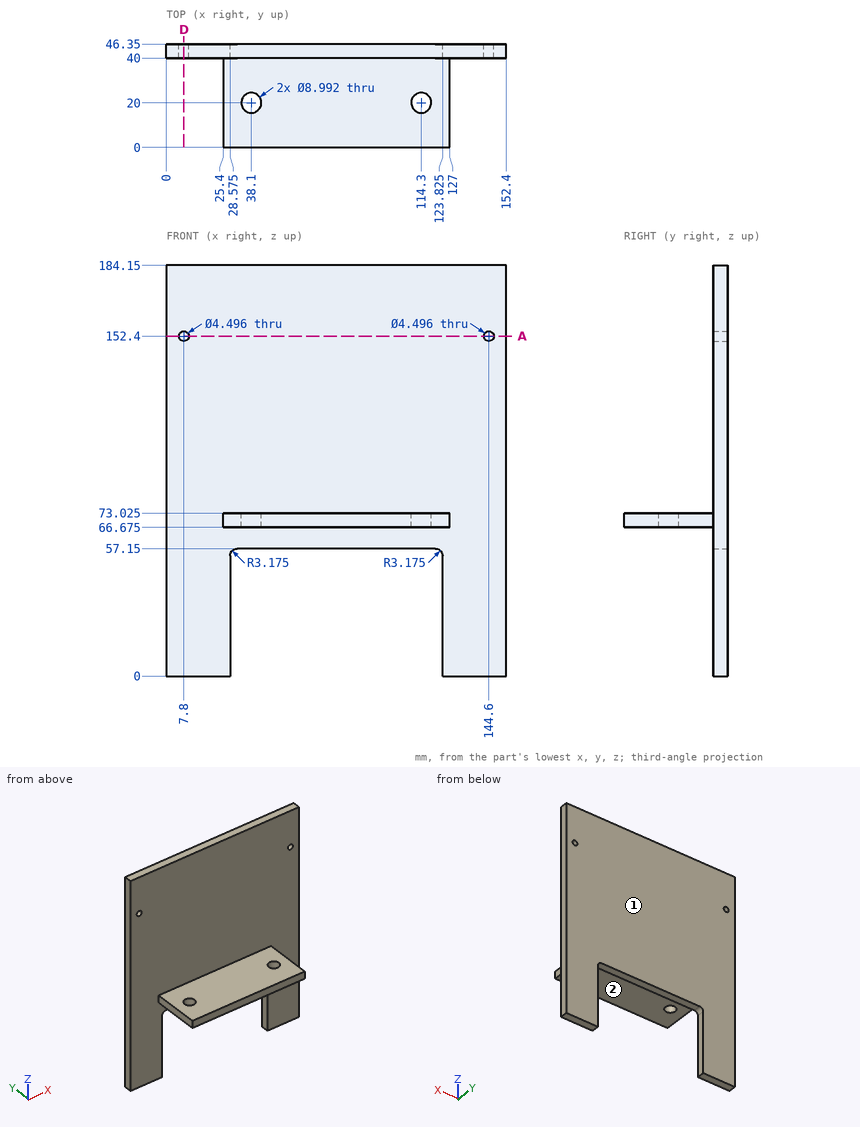
Input: dimensioned drawing with shaded views. Units: mm. Origin: part minimum x, y, z. Give positions to 0.01 mm unless a question says otherwise; leave off trailing zeros. Write each loop counter-clockwise with the first axis right and the second up, starting at its lowest first coordinate (ties: lowest second). Pieces come first, ordered by that corner, then holes.
Q1. First-contact query: P1, Ø7, axis at y = 14.5, z = 70.5, coming from the -X side; P2, Ø10.5, axis at x = 38.1, y = 20, coming from the +Z side (3 decimals); P3, Ø5, axis at y = 27, z = 71, coming from the +X side. Flat tips, straight axial feed; report the tip coordinate or a pass-through.
Q2. Section A-A, the plane z = 152.4. Output: boundary loops of the cut face in (x, y).
Q3. Section D-D, the plane x = 7.8. Output: boundary loops of the cut face in (y, z), plus the area to 3 significant figures.
Q4. Material intervals for probe 1 along X at (y, z) = (20, 71) (1 decimal); probe 2 along X at (y, z) = (41, 152); probe 3 along X at (y, z) = (43, 42) (1 decimal), sorted ascending.
Q5. Pull-direction query (Y, two-part tool) for the marked faces 1 and 2; classes: pulls with the +Y half, pulls with the -Y half, needs draft (parallel to the pull), parting line crosses it, or undercut.
Filled in:
1. P1: stops at x = 25.4
1. P2: stops at z = 73.025
1. P3: stops at x = 127
2. outline: (0, 40) - (5.55, 40) - (5.55, 46.35) - (0, 46.35) - close; (10.05, 40) - (142.35, 40) - (142.35, 46.35) - (10.05, 46.35) - close; (146.85, 40) - (152.4, 40) - (152.4, 46.35) - (146.85, 46.35) - close
3. outline: (40, 0) - (46.35, 0) - (46.35, 150.15) - (40, 150.15) - close; (40, 154.65) - (46.35, 154.65) - (46.35, 184.15) - (40, 184.15) - close
3. area: 1,140 mm2
4. probe 1: x = 25.4 to 33.6, 42.6 to 109.8, 118.8 to 127
4. probe 2: x = 0 to 5.59, 10.01 to 142.39, 146.81 to 152.4
4. probe 3: x = 0 to 28.6, 123.8 to 152.4
5. face 1: pulls with the +Y half
5. face 2: needs draft
